Design review of the part built by this model. Coordinates are the model's own, in mm. Round coordinates to 2 decimals unless told otherwise and drop trailing zeros. Loops run counter-clockwise (first coordinate to the right, second up) from the corner with the lowest first, then second, coordinate; pieces in that order, holes last. Notation, with made-up numbers: (66, 0.25) -> (116, 0.25) arc R6 ccw to (116, 5.25) -> close; hole circle Ø1 at (27, 33). An arc over 180 degrees is marked (long way). Answer as CSV lines item,"result". Start each with the question number.
(1) For P1, Ø5, axis at x = 0, y = 0, coming from the +Z side, flat-tipped, find the tip position at first contact; note if it passes through.
(2) Take a section at C-C, the plane z = -0.25. Write out the cut boundary in (x, y) (1 decimal).
(3) To check wall thickness, follow line 1 (Y direction, x = 0, z = -0.15); line 2 (X direction, y = 2, z = -0.1); line 3 (X direction, y = -0.25, z = -0.2). State the ranges of each line that lie inside material, in increasing order. Write a range as from..to.
(4) Take a section at A-A, the plane x = 0. Write out the cut boundary in (y, z), and give its area (3 significant figures).
from build123d import *

# Parameters (mm, degrees)
SKETCH3_R                = 4.7625
SKETCH3_R_2              = 2.1844
BOSS_EXTRUDE1_DEPTH      = 0.4064
BOSS_EXTRUDE1_DEPTH_BACK = 0.4064
FILLET1_R                = 0.2032


with BuildPart() as part:
    # Sketch3 → Boss-Extrude1 (new body, two sides)
    with BuildSketch(Plane.XY) as boss_extrude1_sk:
        Circle(SKETCH3_R)
        Circle(SKETCH3_R_2, mode=Mode.SUBTRACT)
    extrude(amount=BOSS_EXTRUDE1_DEPTH)
    extrude(boss_extrude1_sk.sketch, amount=-BOSS_EXTRUDE1_DEPTH_BACK)

    # Fillet1
    fillet1_edges = [part.edges().sort_by_distance(p)[0] for p in [
        (-4.7625, 0, 0.4064),
        (-2.1844, 0, 0.4064),
    ]]
    fillet(fillet1_edges, radius=FILLET1_R)


solid = part.part
The answers:
1,P1,"z = 0.41"
2,outline,"circle Ø9.5 at (0, 0); hole circle Ø4.4 at (0, 0)"
3,line 1,"-4.76..-2.18, 2.18..4.76"
3,line 2,"-4.32..-0.88, 0.88..4.32"
3,line 3,"-4.76..-2.17, 2.17..4.76"
4,outline,"(-4.76, -0.41) -> (-2.18, -0.41) -> (-2.18, 0.2) arc R0.2 ccw to (-2.39, 0.41) -> (-4.56, 0.41) arc R0.2 ccw to (-4.76, 0.2) -> close; (2.18, -0.41) -> (4.76, -0.41) -> (4.76, 0.2) arc R0.2 ccw to (4.56, 0.41) -> (2.39, 0.41) arc R0.2 ccw to (2.18, 0.2) -> close"
4,area,"4.16 mm²"
